Input: part model. Units: mm. Frame: model coordinates. Give positions to 0.01 mm unless a question says otherwise; leave off trailing zeros. Loops run counter-clockwise (first coordinate to the right, second up) from the corner with the lowest first, then second, coordinate; pieces in that order, holes last. Notation, with made-up numbers: M 40,-23.5 L 44,-23.5 A14 ccw 44,0.5 Z; hole C -4.5,-22 d7. An arc over 180 degrees is marked long. Answer as a JSON object with one key per item and string values. Group by question number.
```python
from build123d import *

# Parameters (mm, degrees)
F0_W     = 114.3
F0_H     = 266.7
F1_DEPTH = 25.4
F2_R     = 19.05
F2_R_2   = 17.4625
F2_R_3   = 15.875
F2_R_4   = 14.2875
F2_R_5   = 12.7
F2_R_6   = 11.1125
F2_R_7   = 9.525
F2_R_8   = 7.9375
F3_DEPTH = 25.4
F5_DEPTH = 25.4


with BuildPart() as f1:
    # F0 (on Front) → F1 (new body)
    with BuildSketch(Plane.XZ):
        with Locations((-57.15, 133.35)):
            Rectangle(F0_W, F0_H)
    extrude(amount=F1_DEPTH)

    # F2 (on face) → F3 (cut)
    with BuildSketch(Plane.XZ.offset(25.4)):
        with BuildLine():
            ThreePointArc((-25.4, 44.45), (-44.45, 25.4), (-25.4, 6.35))
            Line((-25.4, 6.35), (-25.4, 25.4))
            Line((-25.4, 25.4), (-25.4, 44.45))
        make_face()
        with BuildLine():
            ThreePointArc((-17.4625, 247.65), (-31.01266, 253.26266), (-25.4, 239.7125))
            ThreePointArc((-25.4, 239.7125), (-19.78734, 242.03734), (-17.4625, 247.65))
        make_face()
        with BuildLine():
            ThreePointArc((-25.4, 234.95), (-34.925, 225.425), (-25.4, 215.9))
            Line((-25.4, 215.9), (-25.4, 225.425))
            Line((-25.4, 225.425), (-25.4, 234.95))
        make_face()
        with BuildLine():
            Line((-25.4, 225.425), (-25.4, 215.9))
            ThreePointArc((-25.4, 215.9), (-18.664808, 218.689808), (-15.875, 225.425))
            ThreePointArc((-15.875, 225.425), (-18.664808, 232.160192), (-25.4, 234.95))
            Line((-25.4, 234.95), (-25.4, 225.425))
        make_face()
        with BuildLine():
            ThreePointArc((-25.4, 211.1375), (-36.5125, 200.025), (-25.4, 188.9125))
            Line((-25.4, 188.9125), (-25.4, 200.025))
            Line((-25.4, 200.025), (-25.4, 211.1375))
        make_face()
        with BuildLine():
            Line((-25.4, 200.025), (-25.4, 188.9125))
            ThreePointArc((-25.4, 188.9125), (-17.542276, 192.167276), (-14.2875, 200.025))
            ThreePointArc((-14.2875, 200.025), (-17.542276, 207.882724), (-25.4, 211.1375))
            Line((-25.4, 211.1375), (-25.4, 200.025))
        make_face()
        with BuildLine():
            ThreePointArc((-25.4, 184.15), (-38.1, 171.45), (-25.4, 158.75))
            Line((-25.4, 158.75), (-25.4, 171.45))
            Line((-25.4, 171.45), (-25.4, 184.15))
        make_face()
        with BuildLine():
            Line((-25.4, 171.45), (-25.4, 158.75))
            ThreePointArc((-25.4, 158.75), (-16.419744, 162.469744), (-12.7, 171.45))
            ThreePointArc((-12.7, 171.45), (-16.419744, 180.430256), (-25.4, 184.15))
            Line((-25.4, 184.15), (-25.4, 171.45))
        make_face()
        with BuildLine():
            ThreePointArc((-25.4, 153.9875), (-39.6875, 139.7), (-25.4, 125.4125))
            Line((-25.4, 125.4125), (-25.4, 139.7))
            Line((-25.4, 139.7), (-25.4, 153.9875))
        make_face()
        with BuildLine():
            Line((-25.4, 139.7), (-25.4, 125.4125))
            ThreePointArc((-25.4, 125.4125), (-15.297212, 129.597212), (-11.1125, 139.7))
            ThreePointArc((-11.1125, 139.7), (-15.297212, 149.802788), (-25.4, 153.9875))
            Line((-25.4, 153.9875), (-25.4, 139.7))
        make_face()
        with BuildLine():
            ThreePointArc((-25.4, 120.65), (-41.275, 104.775), (-25.4, 88.9))
            Line((-25.4, 88.9), (-25.4, 104.775))
            Line((-25.4, 104.775), (-25.4, 120.65))
        make_face()
        with BuildLine():
            Line((-25.4, 104.775), (-25.4, 88.9))
            ThreePointArc((-25.4, 88.9), (-14.17468, 93.54968), (-9.525, 104.775))
            ThreePointArc((-9.525, 104.775), (-14.17468, 116.00032), (-25.4, 120.65))
            Line((-25.4, 120.65), (-25.4, 104.775))
        make_face()
        with BuildLine():
            ThreePointArc((-25.4, 84.1375), (-42.8625, 66.675), (-25.4, 49.2125))
            Line((-25.4, 49.2125), (-25.4, 66.675))
            Line((-25.4, 66.675), (-25.4, 84.1375))
        make_face()
        with BuildLine():
            Line((-25.4, 66.675), (-25.4, 49.2125))
            ThreePointArc((-25.4, 49.2125), (-13.052148, 54.327148), (-7.9375, 66.675))
            ThreePointArc((-7.9375, 66.675), (-13.052148, 79.022852), (-25.4, 84.1375))
            Line((-25.4, 84.1375), (-25.4, 66.675))
        make_face()
        with BuildLine():
            Line((-25.4, 25.4), (-25.4, 6.35))
            ThreePointArc((-25.4, 6.35), (-11.929616, 11.929616), (-6.35, 25.4))
            ThreePointArc((-6.35, 25.4), (-11.929616, 38.870384), (-25.4, 44.45))
            Line((-25.4, 44.45), (-25.4, 25.4))
        make_face()
        with Locations((-88.9, 25.4)):
            Circle(F2_R)
        with Locations((-88.9, 66.675)):
            Circle(F2_R_2)
        with Locations((-88.9, 104.775)):
            Circle(F2_R_3)
        with Locations((-88.9, 139.7)):
            Circle(F2_R_4)
        with Locations((-88.9, 171.45)):
            Circle(F2_R_5)
        with Locations((-88.9, 200.025)):
            Circle(F2_R_6)
        with Locations((-88.9, 225.425)):
            Circle(F2_R_7)
        with Locations((-88.9, 247.65)):
            Circle(F2_R_8)
    extrude(amount=-F3_DEPTH, mode=Mode.SUBTRACT)

    # F4 (on face) → F5 (cut)
    with BuildSketch(Plane.XZ.offset(25.4)):
        with BuildLine():
            ThreePointArc((-57.15, 260.35), (-76.2, 241.3), (-57.15, 222.25))
            Line((-57.15, 222.25), (-57.15, 241.3))
            Line((-57.15, 241.3), (-57.15, 260.35))
        make_face()
        with BuildLine():
            Line((-57.15, 241.3), (-57.15, 222.25))
            ThreePointArc((-57.15, 222.25), (-43.679616, 227.829616), (-38.1, 241.3))
            ThreePointArc((-38.1, 241.3), (-43.679616, 254.770384), (-57.15, 260.35))
            Line((-57.15, 260.35), (-57.15, 241.3))
        make_face()
        with BuildLine():
            ThreePointArc((-57.15, 217.4875), (-74.6125, 200.025), (-57.15, 182.5625))
            Line((-57.15, 182.5625), (-57.15, 200.025))
            Line((-57.15, 200.025), (-57.15, 217.4875))
        make_face()
        with BuildLine():
            Line((-57.15, 200.025), (-57.15, 182.5625))
            ThreePointArc((-57.15, 182.5625), (-44.802148, 187.677148), (-39.6875, 200.025))
            ThreePointArc((-39.6875, 200.025), (-44.802148, 212.372852), (-57.15, 217.4875))
            Line((-57.15, 217.4875), (-57.15, 200.025))
        make_face()
        with BuildLine():
            ThreePointArc((-57.15, 177.8), (-73.025, 161.925), (-57.15, 146.05))
            Line((-57.15, 146.05), (-57.15, 161.925))
            Line((-57.15, 161.925), (-57.15, 177.8))
        make_face()
        with BuildLine():
            Line((-57.15, 161.925), (-57.15, 146.05))
            ThreePointArc((-57.15, 146.05), (-45.92468, 150.69968), (-41.275, 161.925))
            ThreePointArc((-41.275, 161.925), (-45.92468, 173.15032), (-57.15, 177.8))
            Line((-57.15, 177.8), (-57.15, 161.925))
        make_face()
        with BuildLine():
            ThreePointArc((-57.15, 141.2875), (-71.4375, 127), (-57.15, 112.7125))
            Line((-57.15, 112.7125), (-57.15, 127))
            Line((-57.15, 127), (-57.15, 141.2875))
        make_face()
        with BuildLine():
            Line((-57.15, 127), (-57.15, 112.7125))
            ThreePointArc((-57.15, 112.7125), (-47.047212, 116.897212), (-42.8625, 127))
            ThreePointArc((-42.8625, 127), (-47.047212, 137.102788), (-57.15, 141.2875))
            Line((-57.15, 141.2875), (-57.15, 127))
        make_face()
        with BuildLine():
            ThreePointArc((-57.15, 107.95), (-69.85, 95.25), (-57.15, 82.55))
            Line((-57.15, 82.55), (-57.15, 95.25))
            Line((-57.15, 95.25), (-57.15, 107.95))
        make_face()
        with BuildLine():
            Line((-57.15, 95.25), (-57.15, 82.55))
            ThreePointArc((-57.15, 82.55), (-48.169744, 86.269744), (-44.45, 95.25))
            ThreePointArc((-44.45, 95.25), (-48.169744, 104.230256), (-57.15, 107.95))
            Line((-57.15, 107.95), (-57.15, 95.25))
        make_face()
        with BuildLine():
            ThreePointArc((-57.15, 77.7875), (-68.2625, 66.675), (-57.15, 55.5625))
            Line((-57.15, 55.5625), (-57.15, 66.675))
            Line((-57.15, 66.675), (-57.15, 77.7875))
        make_face()
        with BuildLine():
            Line((-57.15, 66.675), (-57.15, 55.5625))
            ThreePointArc((-57.15, 55.5625), (-49.292276, 58.817276), (-46.0375, 66.675))
            ThreePointArc((-46.0375, 66.675), (-49.292276, 74.532724), (-57.15, 77.7875))
            Line((-57.15, 77.7875), (-57.15, 66.675))
        make_face()
        with BuildLine():
            ThreePointArc((-57.15, 50.8), (-66.675, 41.275), (-57.15, 31.75))
            Line((-57.15, 31.75), (-57.15, 41.275))
            Line((-57.15, 41.275), (-57.15, 50.8))
        make_face()
        with BuildLine():
            Line((-57.15, 41.275), (-57.15, 31.75))
            ThreePointArc((-57.15, 31.75), (-50.414808, 34.539808), (-47.625, 41.275))
            ThreePointArc((-47.625, 41.275), (-50.414808, 48.010192), (-57.15, 50.8))
            Line((-57.15, 50.8), (-57.15, 41.275))
        make_face()
        with BuildLine():
            ThreePointArc((-49.2125, 19.05), (-51.53734, 24.66266), (-57.15, 26.9875))
            ThreePointArc((-57.15, 26.9875), (-62.76266, 13.43734), (-49.2125, 19.05))
        make_face()
    extrude(amount=-F5_DEPTH, mode=Mode.SUBTRACT)


solid = f1.part
```
1. Section B-B (x = -88.9). Count the separate pieces of the cut face and the enclosed holes in it, then the cut area to 3 significant figures.
2. Section A-A (z = 137). Output: boundary loops of the cut face in (x, y), then the cut area to 3 significant figures.
3. Material intervals for L1, parallel to X at y = -5, z = 219; L2, parallel to X at y = -20, z = 25; L3, parallel to X at y = -1.75, z = 144, sorted ascending.
4. Mould query, pull axis X, two halves, no side actions, for faces 1 (the flat face through (-58, -13, 266.7)), 2 (the flat face through (0, -13, 131)), 3 (the cylindrical face through (-90.62, -12.88, 239.9)). Classes: pulls with the +X half, pulls with the -X half, needs draft (parallel to the pull), parting line crosses it, or undercut.
Geometry results:
{
 "1": {"separate pieces": "9", "enclosed holes": "0", "area": "1,290 mm2"},
 "2": {"outline": "M -114.3,-25.4 L -102.93,-25.4 L -102.93,0 L -114.3,0 Z; M -74.87,-25.4 L -67.35,-25.4 L -67.35,0 L -74.87,0 Z; M -46.95,-25.4 L -39.43,-25.4 L -39.43,0 L -46.95,0 Z; M -11.37,-25.4 L 0,-25.4 L 0,0 L -11.37,0 Z", "area": "959 mm2"},
 "3": {"L1": "-114.3 to -95.93, -81.87 to -32.43, -18.37 to 0", "L2": "-114.3 to -107.95, -69.85 to -62.4, -51.9 to -44.45, -6.35 to 0", "L3": "-114.3 to -102.53, -75.27 to -39.03, -11.77 to 0"},
 "4": {"face 1": "needs draft", "face 2": "pulls with the +X half", "face 3": "undercut"}
}
